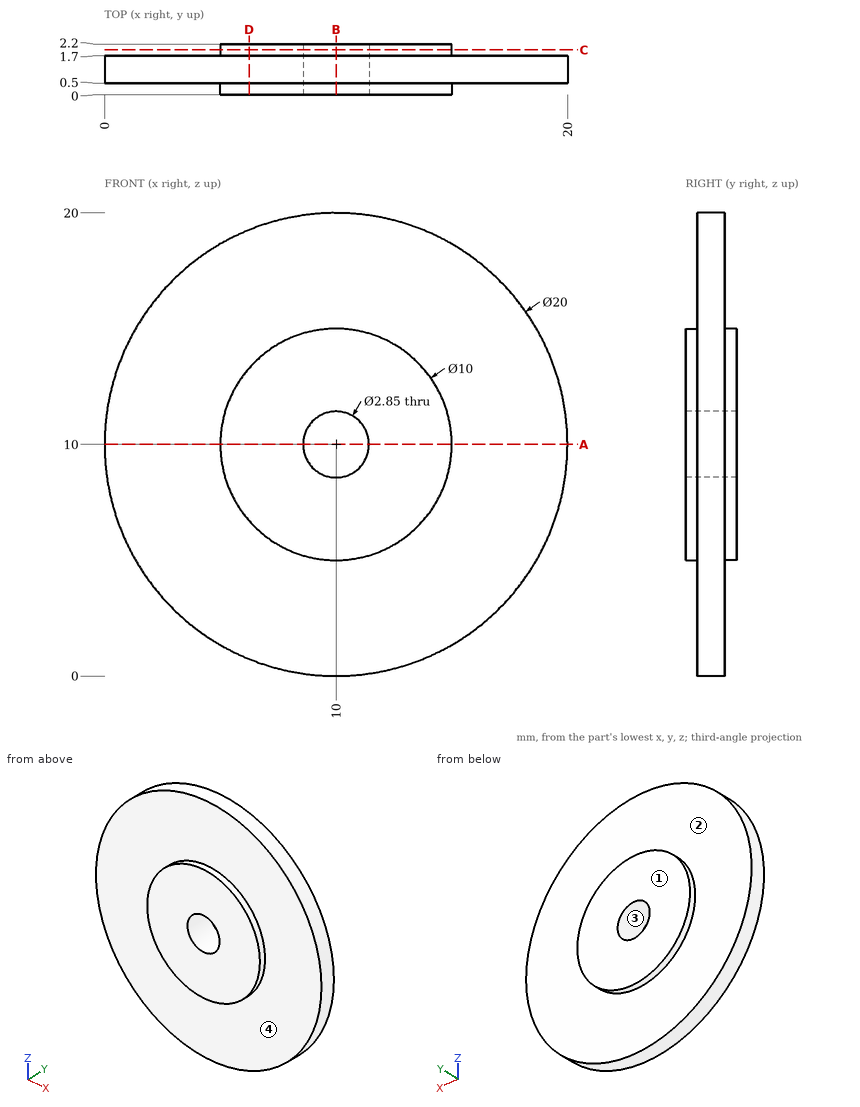
Geometry: see drawing. Coordinates: mm, zero at the bounding-box minimum. A direction names the side the tool comes from. Coordinates: 2 decimals unless noted, no trailing zeros. Write each loop counter-clockwise with the first axis right and the second up, starting at its lowest first coordinate (ties: lowest second). Pieces come first, ordered by that corner, then holes. Notation, with made-up numbers: M -23.5,42 L 31.5,42 A17 ccw 31.5,75 Z; hole C 52.5,-30 d2. An arc over 180 degrees is marked long. Use CSV: the item, a comma, the result in double quotes. Start each with the question number.
1. Ray query, probe 1 along Z at (x, y) = (10, 0.6) (3 decimals); probe 2 along Z at (x, y) = (10, 0.45) (3 decimals); probe 3 along Y at (x, z) = (3.25, 7.75). Return the intervals inside material, ascending.
2. Cut plane A-A on z = 10. Return the cut outline in (x, y) (3 decimals), plus the area to 3 significant figures.
3. Cut plane C-C on y = 1.95. Return the cut outline in (x, z) (3 decimals), plus the area to 3 significant figures.
4. Reachability of the marked faces 1 and 2 from +Z, -Z, +X, -X, +Y, -Y: full face, straight path, thin tool, end or side. Return the list, or none.
5. Cut plane D-D on x = 6.25. Return the cut outline in (y, z).
6. First-contact query: P1, Ø6, axis at x = 12, z = 11, coming from the -Y side; P2, Ø8, axis at x = 16, z = 17, coming from the -Y side; P3, Ø1, axis at y = 1.5, z = 8.5, coming from the -X side. Flat tips, straight axial feed; report the tip coordinate or a pass-through.
7. Cut plane B-B on x = 10. Return the cut outline in (y, z) (3 decimals), plus the area to 3 significant figures.
8. Mould query, pull axis Z, two halves, no side actions, for the marked faces 3 and 4. Classes: pulls with the +Z half, pulls with the -Z half, needs draft (parallel to the pull), parting line crosses it, or undercut.
Entries:
1,probe 1,"0 to 8.575, 11.425 to 20"
1,probe 2,"5 to 8.575, 11.425 to 15"
1,probe 3,"0.5 to 1.7"
2,outline,"M 0,0.5 L 5,0.5 L 5,0 L 8.575,0 L 8.575,2.2 L 5,2.2 L 5,1.7 L 0,1.7 Z; M 11.425,0 L 15,0 L 15,0.5 L 20,0.5 L 20,1.7 L 15,1.7 L 15,2.2 L 11.425,2.2 Z"
2,area,"27.7 mm²"
3,outline,"C 10,10 d10; hole C 10,10 d2.85"
3,area,"72.2 mm²"
4,face 1,"+Z, -Z, +X, -X, +Y"
4,face 2,"+Y"
5,outline,"M 0,6.69 L 0.5,6.69 L 0.5,0.73 L 1.7,0.73 L 1.7,6.69 L 2.2,6.69 L 2.2,13.31 L 1.7,13.31 L 1.7,19.27 L 0.5,19.27 L 0.5,13.31 L 0,13.31 Z"
6,P1,"y = 0"
6,P2,"y = 0.5"
6,P3,"x = 0.05"
7,outline,"M 0,5 L 0.5,5 L 0.5,0 L 1.7,0 L 1.7,5 L 2.2,5 L 2.2,8.575 L 0,8.575 Z; M 0,11.425 L 2.2,11.425 L 2.2,15 L 1.7,15 L 1.7,20 L 0.5,20 L 0.5,15 L 0,15 Z"
7,area,"27.7 mm²"
8,face 3,"undercut"
8,face 4,"needs draft"
